CAD build for the part. Positions are in the model's coordinates, mm. A direction names the side the tool comes from. Give positions to 0.01 mm unless a question says otherwise; leave off trailing zeros. Order: outer loops, then holes, each group sorted by start corner. A loop starts at its lowest first (then second) coordinate and runs counter-clockwise, first axis right, second up.
from build123d import *

# Parameters (mm, degrees)
F1_DEPTH = 92.71
F3_DEPTH = 33.528
F4_R     = 21.401404
F5_DEPTH = 42.164


with BuildPart() as f1:
    # F0 (on Top) → F1 (new body)
    with BuildSketch(Plane.XY):
        Polygon((19.526986, 33.821732), (-19.526986, 33.821732), (-39.053972, 0), (-19.526986, -33.821732), (19.526986, -33.821732), (39.053972, 0), align=None)
    extrude(amount=F1_DEPTH)

    # F2 (on face) → F3 (join)
    with BuildSketch(Plane.XY.offset(92.71)):
        Polygon((10.06457, 17.432347), (-10.06457, 17.432347), (-20.12914, 0), (-10.06457, -17.432347), (10.06457, -17.432347), (20.12914, 0), align=None)
    extrude(amount=F3_DEPTH)

    # F4 (on face) → F5 (join)
    with BuildSketch(Plane(origin=(0, 0, 0), x_dir=(1, 0, 0), z_dir=(0, 0, -1))):
        Circle(F4_R)
    extrude(amount=F5_DEPTH)


solid = f1.part
1. Saw through at D-D on z = 83.5. Give the cut face in (x, y), plus the area to 3 significant figures.
2. 3-axis set-ups, long thin cutter, end or side, ignore diameter. For faces 1 (the flat face through (0, 17.432, 109)), 2 (the flat face through (0, -17.432, 109)), 3 (the flat face through (-15.17, -8.59, 109.24)), 4 (the flat face through (-15.026, 8.838, 109.239)), 5 (the flat face through (17, 16, 0)): which of +Z, -Z, +X, -X, +Y, -Y reach the whole face in a straight line?
3. Saw through at B-B on z = 107. Give the cut face in (x, y), plus the area to 3 significant figures.
4. Pin check, flat tips, straight feed: P1, Ø12, axis at y = 18.5, z = 37.5, coming from the +X side; P2, Ø6, axis at x = 6, y = -24, coming from the +Z side; P3, Ø22, axis at x = -1, z = 110.5, coming from the -Y side. Stop position of each tip, or through.
5. Saw through at C-C on y = 7.5. Give the cut face in (x, z), plus the area to 3 significant figures.
6. Saw through at A-A on x = 0. Give the cut face in (y, z).
7. Wall check: line 1 (Z direction, x = 2, y = -23); line 2 (X direction, y = 3, z = 2); line 3 (Y direction, x = -32, z = 87). Give the ranges that are in metal, low to high.
Reported:
1. outline: (-39.05, 0) - (-19.53, -33.82) - (19.53, -33.82) - (39.05, 0) - (19.53, 33.82) - (-19.53, 33.82) - close
1. area: 3,960 mm2
2. face 1: +Z, +X, -X, +Y
2. face 2: +Z, +X, -X, -Y
2. face 3: +Z, -X, -Y
2. face 4: +Z, -X, +Y
2. face 5: -Z
3. outline: (-20.13, 0) - (-10.06, -17.43) - (10.06, -17.43) - (20.13, 0) - (10.06, 17.43) - (-10.06, 17.43) - close
3. area: 1,050 mm2
4. P1: stops at x = 31.84
4. P2: stops at z = 92.71
4. P3: stops at y = -17.43
5. outline: (-34.72, 0) - (-20.04, 0) - (-20.04, -42.16) - (20.04, -42.16) - (20.04, 0) - (34.72, 0) - (34.72, 92.71) - (15.8, 92.71) - (15.8, 126.24) - (-15.8, 126.24) - (-15.8, 92.71) - (-34.72, 92.71) - close
5. area: 9,190 mm2
6. outline: (-33.82, 0) - (-21.4, 0) - (-21.4, -42.16) - (21.4, -42.16) - (21.4, 0) - (33.82, 0) - (33.82, 92.71) - (17.43, 92.71) - (17.43, 126.24) - (-17.43, 126.24) - (-17.43, 92.71) - (-33.82, 92.71) - close
7. line 1: z = 0 to 92.71
7. line 2: x = -37.32 to 37.32
7. line 3: y = -12.22 to 12.22
